from build123d import *

# Parameters (mm, degrees)
BOSS_EXTRUDE1_DEPTH = 5.588


with BuildPart() as part:
    # Sketch1 → Boss-Extrude1 (new body)
    with BuildSketch(Plane(origin=(-5.329574036, -16.20301374, 0), x_dir=(1, 0, 0), z_dir=(0, 0, 1))):
        Polygon((-288.637525151, -72.531124316), (-294.987525151, -72.531124316), (-294.987525151, -90.311124316), (-288.637525151, -90.311124316), (-288.637525151, -115.711124316), (-294.987525151, -115.711124316), (-294.987525151, -133.491124316), (-288.637525151, -133.491124316), (-288.637525151, -165.241124316), (-263.237525151, -165.241124316), (-263.237525151, -158.891124316), (-237.837525151, -158.891124316), (-237.837525151, -165.241124316), (-212.437525151, -165.241124316), (-212.437525151, -158.891124316), (-187.037525151, -158.891124316), (-187.037525151, -165.241124316), (-161.637525151, -165.241124316), (-161.637525151, -158.891124316), (-136.237525151, -158.891124316), (-136.237525151, -165.241124316), (-110.837525151, -165.241124316), (-110.837525151, -158.891124316), (-85.437525151, -158.891124316), (-85.437525151, -165.241124316), (-60.037525151, -165.241124316), (-60.037525151, -158.891124316), (-34.637525151, -158.891124316), (-34.637525151, -165.241124316), (-9.237525151, -165.241124316), (-9.237525151, -158.891124316), (16.162474849, -158.891124316), (16.162474849, -133.491124316), (21.632687755, -133.491124316), (21.632687755, -115.711124316), (16.162474849, -115.711124316), (16.162474849, -90.311124316), (21.632687755, -90.311124316), (21.632687755, -72.531124316), (16.162474849, -72.531124316), (16.162474849, -40.781124316), (-9.237525151, -40.781124316), (-9.237525151, -47.131124316), (-34.637525151, -47.131124316), (-34.637525151, -40.781124316), (-60.037525151, -40.781124316), (-60.037525151, -47.131124316), (-85.437525151, -47.131124316), (-85.437525151, -40.781124316), (-110.837525151, -40.781124316), (-110.837525151, -47.131124316), (-139.412525151, -47.131124316), (-139.412525151, -40.781124316), (-161.637525151, -40.781124316), (-161.637525151, -47.131124316), (-187.037525151, -47.131124316), (-187.037525151, -40.781124316), (-212.437525151, -40.781124316), (-212.437525151, -47.131124316), (-237.837525151, -47.131124316), (-237.837525151, -40.781124316), (-263.237525151, -40.781124316), (-263.237525151, -47.131124316), (-288.637525151, -47.131124316), align=None)
    extrude(amount=BOSS_EXTRUDE1_DEPTH)


solid = part.part
Can you work these out from the model? Positions are in its coordinate system, mm. A direction names the side the tool comes from. Coordinates: 2 decimals unless noted, no trailing zeros. Write each loop counter-clockwise with the first axis right and the second up, starting at its lowest first coordinate (ties: lowest second). Pieces come first, ordered by that corner, then holes. Notation, with made-up numbers: (-7, 49.25) - (39, 49.25) arc R18 cw to (39, 72.25) - close; hole circle Ø8 at (-38, 56.25). An arc over 180 degrees is marked (long way). Return JSON: item names as keys, results as strings. Group by question number.
Item 1: I'm going to push flat-ended pins straight in: pin 1 Ø3 at (y, z) = (-61, 3.5) entering from +X; pin 2 Ø3 at (x, z) = (-239.5, 5) entering from +Y; pin 3 Ø1.6 at (x, z) = (14.5, 3) entering from -Y. Where does each tip first touch, or does it pass through?
Item 2: We'd pull the mould along X, two halves only. Please class faces 1 (the face through (-78, -63.334, 3)), 2 (the face through (14, -131.914, 3)), 3 (the face through (-14.567, -178, 3)), 4 (the face through (-300.317, -97, 3)): pulls with the +X half, pulls with the -X half, needs draft (parallel to the pull), parting line crosses it, or undercut.
Item 3: If we section it at B-B (y = -79): Write out the boundary of the cut face in (x, z).
Item 4: Please list where these lines run through material, in increasing order: probe 1 along X at (y, z) = (-175.5, 2.75); probe 2 along Y at (x, z) = (-51, 0.4); probe 3 along Y at (x, z) = (-231.5, 4.15).
Item 5: Which directions (+Z, -Z, +X, -X, +Y, -Y) give clear straight access to the entire face, cutting with the end or side of a thin tool? Please do faces 5 (the face through (10.833, -163, 3)), 6 (the face through (-217.767, -178, 3)), 7 (the face through (-27, -63.334, 3)), 8 (the face through (10.833, -119, 3)).
Item 6: If we section it at A-A (x = -197.5): Write out the boundary of the cut face in (y, z).
Return value:
{
 "1": {"pin 1": "stops at x = 10.83", "pin 2": "stops at y = -63.33", "pin 3": "stops at y = -149.69"},
 "2": {"face 1": "undercut", "face 2": "needs draft", "face 3": "pulls with the +X half", "face 4": "pulls with the -X half"},
 "3": {"outline": "(-293.97, 0) - (10.83, 0) - (10.83, 5.59) - (-293.97, 5.59) - close"},
 "4": {"probe 1": "x = -293.97 to -268.57, -243.17 to -217.77, -192.37 to -166.97, -141.57 to -116.17, -90.77 to -65.37, -39.97 to -14.57", "probe 2": "y = -175.09 to -56.98", "probe 3": "y = -181.44 to -63.33"},
 "5": {"face 5": "+Z, -Z, +X, -Y", "face 6": "+Z, -Z, -Y", "face 7": "+Z, -Z, +Y", "face 8": "+Z, -Z, +X"},
 "6": {"outline": "(-175.09, 0) - (-56.98, 0) - (-56.98, 5.59) - (-175.09, 5.59) - close"}
}
